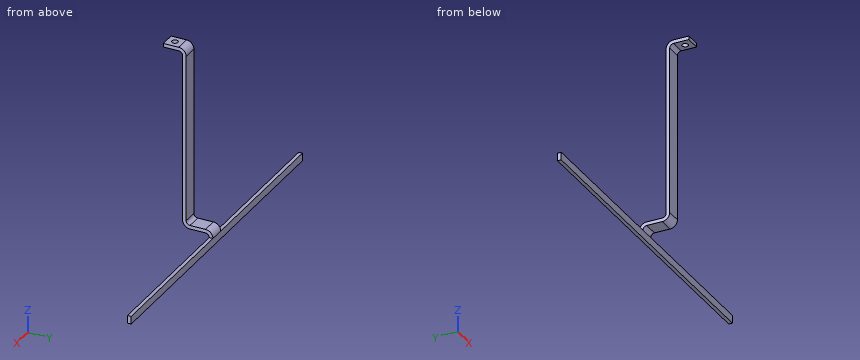
Autodesk Inventor part; units mm, degrees
ref_plane "YZ Plane" through (0, 0, 0) normal (1, 0, 0) x (0, 1, 0)
ref_plane "XZ Plane" through (0, 0, 0) normal (0, 1, 0) x (-1, 0, 0)
ref_plane "XY Plane" through (0, 0, 0) normal (0, 0, 1) x (1, 0, 0)
sketch "Sketch1" plane through (0, 0, 0) normal (0, 0, 1) x (1, 0, 0)
  line L0 (0, 0) -> (-12.7, 0)
  line L1 (-12.7, 0) -> (-12.7, 19.05)
  line L2 (-12.7, 19.05) -> (0, 19.05)
  line L3 (0, 19.05) -> (0, 0)
  dimension "d0" = 12.7
  dimension "d1" = 19.05
extrude "Plate1" add sketch "Sketch1" along normal blind 3.048
sketch "Sketch2" plane through (0, 16.002, 3.048) normal (0, 1, 0) x (-1, 0, 0)
  line L0 (12.7, 0) -> (0, 0)
  line L1 (0, 0) -> (0, -152.4)
  line L2 (0, -152.4) -> (12.7, -152.4)
  line L3 (12.7, -152.4) -> (12.7, 0)
edge flange "Flange1" height 152.4 angle 90 thickness 3.048 bend radius 3.175 thickness toward (0, 1, 0) relief tear relief width 3.048 relief depth 1.524 edges at (-6.35, 19.05, 0) wall of the first edge with corners at (-12.7, 16.002, 3.048) (0, 16.002, 3.048) (0, 16.002, -149.352) (-12.7, 16.002, -149.352)
bend "Bend1"
corner "Corner1"
sketch "Sketch3" plane through (0, 0, 3.048) normal (0, 0, 1) x (1, 0, 0)
  line L0 (0, 12.827) -> (-12.7, 12.827)
  line L1 (0, 12.827) -> (0, 0)
  circle A0 centre (-6.35, 6.4135) radius 2.54
  dimension "d13" = 5.08
  dimension "d15" = 6.4135
  dimension "d16" = 6.35
extrude "Cut1" cut sketch "Sketch3" against normal blind 3.048
sketch "Sketch4" plane through (-12.7, 16.002, -146.304) normal (0, 0, -1) x (-1, 0, 0)
  line L0 (-12.7, 0) -> (0, 0)
  line L1 (0, 0) -> (0, 25.4)
  line L2 (0, 25.4) -> (-12.7, 25.4)
  line L3 (-12.7, 25.4) -> (-12.7, 0)
edge flange "Flange2" height 25.4 angle 90 thickness 3.048 bend radius 3.175 thickness toward (0, 0, -1) relief tear relief width 3.048 relief depth 1.524 edges at (-6.35, 19.05, -149.352) wall of the first edge with corners at (0, 16.002, -146.304) (-12.7, 16.002, -146.304) (-12.7, 41.402, -146.304) (0, 41.402, -146.304)
bend "Bend2"
corner "Corner2"
sketch "Sketch5" plane through (0, 38.354, -146.304) normal (0, 1, 0) x (-1, 0, 0)
  line L0 (12.7, 0) -> (0, 0)
  line L1 (0, 0) -> (0, -12.7)
  line L2 (0, -12.7) -> (12.7, -12.7)
  line L3 (12.7, -12.7) -> (12.7, 0)
edge flange "Flange3" height 12.7 angle 90 thickness 3.048 bend radius 3.175 thickness toward (0, 1, 0) relief tear relief width 3.048 relief depth 1.524 edges at (-6.35, 41.402, -149.352) wall of the first edge with corners at (-12.7, 38.354, -146.304) (0, 38.354, -146.304) (0, 38.354, -159.004) (-12.7, 38.354, -159.004)
bend "Bend3"
corner "Corner3"
sketch "Sketch6" plane through (0, 38.354, -159.004) normal (1, 0, 0) x (0, 0, -1)
  line L0 (-6.477, 3.048) -> (-6.477, 0)
  line L1 (0, 0) -> (-6.477, 0)
  line L2 (0, 0) -> (0, 3.048)
  line L3 (0, 3.048) -> (-6.477, 3.048)
  point P0 (-159.004, -38.354)
extrude "Extrusion1" add sketch "Sketch6" along normal blind 133.35
sketch "Sketch7" plane through (-12.7, 38.354, -159.004) normal (-1, 0, 0) x (0, 0, 1)
  line L0 (6.477, 0) -> (6.477, 3.048)
  line L1 (6.477, 3.048) -> (0, 3.048)
  line L2 (0, 0) -> (0, 3.048)
  line L3 (0, 0) -> (6.477, 0)
  point P0 (159.004, -38.354)
extrude "Extrusion2" add sketch "Sketch7" along normal blind 133.35
sketch "Sketch8" plane through (0, 16.002, -3.175) normal (1, 0, 0) x (0, 0, -1)
  line L0 (139.954, 0) -> (139.954, 3.048)
  line L1 (139.954, 3.048) -> (0, 3.048)
  line L2 (0, 3.048) -> (0, 0)
  line L3 (139.954, 0) -> (0, 0)
  line L4 (12.7, 3.048) -> (25.4, 3.048)
  line L5 (25.4, 3.048) -> (25.4, 0)
  line L6 (25.4, 0) -> (12.7, 0)
  line L7 (12.7, 3.048) -> (12.7, 0)
  point P0 (-3.175, -16.002)
  dimension "d43" = 12.7
  dimension "d44" = 12.7
sketch "Sketch9" plane through (0, 38.354, -152.527) normal (0, 0, 1) x (1, 0, 0)
  line L0 (0, 3.048) -> (0, 0)
  line L1 (0, 0) -> (133.35, 0)
  line L2 (133.35, 3.048) -> (133.35, 0)
  line L3 (0, 3.048) -> (133.35, 3.048)
  line L4 (133.35, 0) -> (120.65, 0)
  line L5 (120.65, 0) -> (120.65, 3.048)
  line L6 (133.35, 3.048) -> (120.65, 3.048)
  line L7 (133.35, 3.048) -> (133.35, 0)
  point P0 (0, -38.354)
  dimension "d45" = 12.7
equation "\"d17\" = Thickness"
equation "\"d3\" = BendReliefWidth"
equation "\"d4\" = BendReliefDepth"
equation "\"d5\" = MinimumRemnant"
equation "\"d6\" = BendRadius"
equation "\"d10\" = CornerReliefSize"
equation "\"d11\" = GapSize"
equation "\"d12\" = JacobiRadiusSize"
equation "\"d19\" = BendReliefWidth"
equation "\"d20\" = BendReliefDepth"
equation "\"d21\" = MinimumRemnant"
equation "\"d22\" = BendRadius"
equation "\"d26\" = CornerReliefSize"
equation "\"d27\" = GapSize"
equation "\"d28\" = JacobiRadiusSize"
equation "\"d29\" = BendReliefWidth"
equation "\"d30\" = BendReliefDepth"
equation "\"d31\" = MinimumRemnant"
equation "\"d32\" = BendRadius"
equation "\"d36\" = CornerReliefSize"
equation "\"d37\" = GapSize"
equation "\"d38\" = JacobiRadiusSize"
equation "\"BendRadius\" = Thickness"
equation "\"BendReliefWidth\" = Thickness"
equation "\"BendReliefDepth\" = 0.5 * Thickness"
equation "\"CornerReliefSize\" = 4 * Thickness"
equation "\"MinimumRemnant\" = 2 * Thickness"
equation "\"TransitionRadius\" = BendRadius"
equation "\"JacobiRadiusSize\" = BendRadius"
equation "\"GapSize\" = Thickness"
equation "\"d2\" = BendRadius"
properties part number "Feeder-Grabber_v1"
The listing builds one solid part. Answer for the finished solid, in the listing's coordinates (mm). Coordinates: 2 decimals unless noted, no trailing zeros. Loops run counter-clockwise (first coordinate to the right, second up) from the corner with the lowest first, then second, coordinate; pieces in that order, holes last. Notation, with made-up numbers: (82, 75.25) -> (107, 75.25) arc R16 cw to (107, 104.25) -> close; hole circle Ø8 at (67, -36). An arc over 180 degrees is marked (long way). Answer in a Markdown table with one row per item. Add a question column.
1. The part is cut by section A-A, the plane x = -72. Write down the section's boundary in (y, z).
2. Consider line 1 (Y direction, x = -6.35, z = 2.2); line 2 (X direction, y = 19, z = -136); line 3 (Y direction, x = -6.35, z = 1.65). Determine where each line is inside the solid, lowest interval first. Write a range as [from, to].
3. Flat-ended cylindrical pins translate along their axes: P1, Ø4, axis at x = -4, y = 28, coming from the -Z side; P2, Ø6.5, axis at x = -7.5, z = -87.5, coming from the -Y side; P3, Ø1.5, axis at x = -96, y = 40, coming from the +Z side. Find the tip coordinate at first contact, or state that the pin passes through.
4. The part is cut by section B-B, the plane y = 31. Write down the section's boundary in (x, z).
Answer below:
| question | item | result |
|---|---|---|
| 1 | outline | (38.35, -159) -> (41.4, -159) -> (41.4, -152.53) -> (38.35, -152.53) -> close |
| 2 | line 1 | [0, 3.87], [8.95, 15.96] |
| 2 | line 2 | [-12.7, 0] |
| 2 | line 3 | [0, 3.87], [8.95, 16.76] |
| 3 | P1 | z = -149.35 |
| 3 | P2 | y = 16 |
| 3 | P3 | z = -152.53 |
| 4 | outline | (-12.7, -149.35) -> (0, -149.35) -> (0, -146.3) -> (-12.7, -146.3) -> close |
